```python
from build123d import *

# Parameters (mm, degrees)
SKETCH1_R           = 33
BOSS_EXTRUDE1_DEPTH = 5
CUT_EXTRUDE3_START  = -10
CUT_EXTRUDE3_DEPTH  = 10
FILLET2_R           = 20
FILLET3_R           = 15
SKETCH7_W           = 5
SKETCH7_H           = 5
SKETCH7_W_2         = 7
CUT_EXTRUDE4_DEPTH  = 10
SKETCH8_W           = 10
SKETCH8_H           = 7
CUT_EXTRUDE5_DEPTH  = 10


with BuildPart() as part:
    # Sketch1 → Boss-Extrude1 (new body)
    with BuildSketch(Plane.XY):
        Circle(SKETCH1_R)
    extrude(amount=BOSS_EXTRUDE1_DEPTH)

    # Sketch6 → Cut-Extrude3 (cut)
    with BuildSketch(Plane.XY.offset(5).offset(CUT_EXTRUDE3_START)):
        with BuildLine():
            Line((-20, 26.248809497), (-20, -26.248809497))
            ThreePointArc((-20, -26.248809497), (-33, 0), (-20, 26.248809497))
        make_face()
        with BuildLine():
            Line((20, -26.248809497), (20, 26.248809497))
            ThreePointArc((20, 26.248809497), (33, 0), (20, -26.248809497))
        make_face()
    extrude(amount=CUT_EXTRUDE3_DEPTH, mode=Mode.SUBTRACT)

    # Fillet2
    fillet2_edges = [part.edges().sort_by_distance(p)[0] for p in [
        (-20, 26.248809497, 2.5),
        (20, 26.248809497, 2.5),
    ]]
    fillet(fillet2_edges, radius=FILLET2_R - 0.0001)  # a hair under: the kernel refuses the full size

    # Fillet3
    fillet3_edges = [part.edges().sort_by_distance(p)[0] for p in [
        (-20, -26.248809497, 2.5),
        (20, -26.248809497, 2.5),
    ]]
    fillet(fillet3_edges, radius=FILLET3_R)

    # Sketch7 → Cut-Extrude4 (cut)
    with BuildSketch(Plane.XY.offset(5)):
        with Locations((0, 24)):
            Rectangle(SKETCH7_W, SKETCH7_H)
        with Locations((0, -23.5)):
            Rectangle(SKETCH7_W_2, SKETCH7_H)
    extrude(amount=-CUT_EXTRUDE4_DEPTH, mode=Mode.SUBTRACT)

    # Sketch8 → Cut-Extrude5 (cut)
    with BuildSketch(Plane.XY.offset(5)):
        with Locations((10, -9)):
            Rectangle(SKETCH8_W, SKETCH8_H)
    extrude(amount=-CUT_EXTRUDE5_DEPTH, mode=Mode.SUBTRACT)


solid = part.part
```
Geometry: final body of the model. Coordinates: model frame, mm. A direction names the side the tool comes from. Coordinates: 2 decimals unless noted, no trailing zeros. Order: outer loops, then holes, each group sorted by start corner. A loop starts at its lowest first (then second) coordinate and runs counter-clockwise, first axis right, second up. Notation, with made-up numbers: M 25,56.5 L 82,56.5 A16 ccw 82,73.5 Z; hole C -38,4 d6. An arc over 180 degrees is marked long. Answer in a Markdown table with one row per item. Add a question column.
Q1. Line query: L1, parallel to Y at x = -0.5, z = 3; L2, parallel to X at y = -8, z = 3.25; L3, parallel to Y at x = 13, z = 2.6. Output: solid intervals per line, ascending.
Q2. Section query D-D on x = -1.5. Return the cut outline in (y, z), and give its area (3 significant figures).
Q3. Mould query, pull axis X, two halves, no side actions, for faces 1 (the cylindrical face through (-16.91, -26.41, 2.54)), 2 (the cylindrical face through (0, -33, 2)), 3 (the flat face through (10, -5.5, 3)). Classes: released by +X, released by -X, zero draft, split by the parting line, or undercut.
Q4. Section query C-C on x = 10.5. Return the cut outline in (y, z).
Q5. Section query B-B on y = -22.5. Return the cut outline in (x, z).
Q6. Section query A-A on z = 3.2. Count the separate pieces of the cut face and the enclosed holes in it, and give its area (3 significant figures).
Q7. Contact query for flat-ended pins moving along their axis: P1, Ø1.5, axis at y = -25.5, z = 2.5, coming from the +X side; P2, Ø2.5, axis at y = 25, z = 1.5, coming from the +X side; P3, Ø2.5, axis at x = -0.5, z = 2, coming from the -Y side. Output: stop coordinate, or through.
Q8. Reachability of faces 4 (the flat face through (0, 21.5, 3)), 5 (the flat face through (0, 0, 5)) from +Z, -Z, +X, -X, +Y, -Y: full face, straight path, thin tool, end or side. Return the list, or none.
Completed:
| question | item | result |
|---|---|---|
| 1 | L1 | y = -33 to -26, -21 to 21.5, 26.5 to 32.99 |
| 1 | L2 | x = -20 to 5, 15 to 20 |
| 1 | L3 | y = -29.98 to -12.5, -5.5 to 28.2 |
| 2 | outline | M -32.97,0 L -26,0 L -26,5 L -32.97,5 Z; M -21,0 L 21.5,0 L 21.5,5 L -21,5 Z; M 26.5,0 L 32.94,0 L 32.94,5 L 26.5,5 Z |
| 2 | area | 280 mm2 |
| 3 | face 1 | released by -X |
| 3 | face 2 | split by the parting line |
| 3 | face 3 | undercut |
| 4 | outline | M -31.25,0 L -12.5,0 L -12.5,5 L -31.25,5 Z; M -5.5,0 L 30.02,0 L 30.02,5 L -5.5,5 Z |
| 5 | outline | M -19.07,0 L -3.5,0 L -3.5,5 L -19.07,5 Z; M 3.5,0 L 19.07,0 L 19.07,5 L 3.5,5 Z |
| 6 | separate pieces | 1 |
| 6 | enclosed holes | 3 |
| 6 | area | 2,220 mm2 |
| 7 | P1 | stops at x = 18.01 |
| 7 | P2 | stops at x = 16.87 |
| 7 | P3 | stops at y = -33 |
| 8 | face 4 | +Z, -Z |
| 8 | face 5 | +Z, +X, -X, +Y, -Y |
